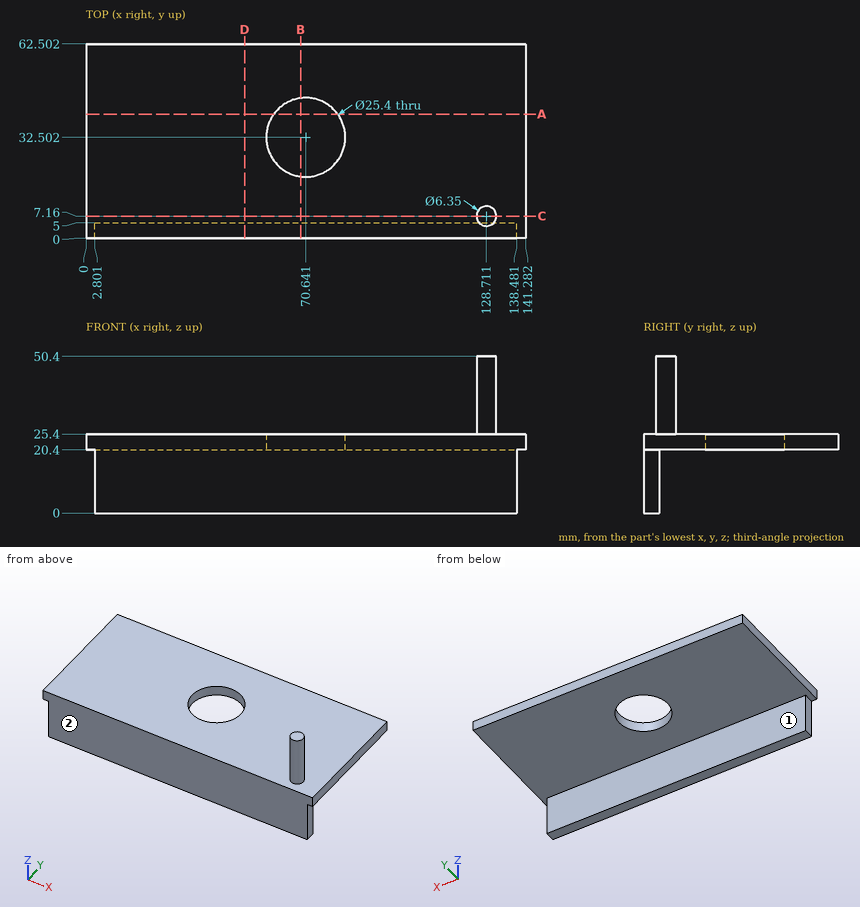
Design review of the part shown in the three views and the two pictorial views. Dimensions are in mm from the part's minimum x, y and z. A direction names the side the tool comes from. Round coordinates to 2 decimals unless told otherwise and drop trailing zeros. Order: outer loops, then holes, each group sorted by start corner. A loop starts at its lowest first (then second) coordinate and runs counter-clockwise, first axis right, second up.
Q1. Insertion check: P1, Ø6, axis at x = 41.5, z = 8, coming from the +Y side; P2, Ø1.5, axis at x = 45, y = 11.5, coming from the -Z side; P3, Ø5, axis at y = 22, z = 29.5, coming from the +X side; P4, Ø1, axis at x = 103, y = 35.5, coming from the +Z side. Each pin has a flat end and moves straight along its axis. Give the tip position at first contact, or say it passes through.
Findings below:
P1: stops at y = 5
P2: stops at z = 20.4
P3: passes through
P4: stops at z = 25.4
Q2. Machinability: for the marked faces 1 and 2, which of the approach directions +Z, -Z, +X, -X, +Y, -Y give a long, thin tool a straight path to every point of the face, cutting with its end or side? Answer none if there is none.
Findings below:
face 1: -Z, +X, -X, +Y
face 2: +Z, -Z, +X, -X, -Y
Q3. Wall thickness on line 1 (Z direction, x = 60.5, y = 41.5); line 2 (Y direction, x = 131.5, z = 15.5); line 3 (X direction, y = 24, z = 22.5) (1 decimal): over which ranges is each line inside the solid? List them lowest first.
Findings below:
line 1: z = 20.4 to 25.4
line 2: y = 0 to 5
line 3: x = 0 to 61.2, 80.1 to 141.3
Q4. We need section A-A, the plane y = 40. Give the boundary of the cut face in (x, z), plus the area to 3 significant figures.
Findings below:
outline: (0, 20.4) - (60.39, 20.4) - (60.39, 25.4) - (0, 25.4) - close; (80.89, 20.4) - (141.28, 20.4) - (141.28, 25.4) - (80.89, 25.4) - close
area: 604 mm2
Q5. We need section B-B, the plane x = 69. Give the boundary of the cut face in (y, z).
Findings below:
outline: (0, 0) - (5, 0) - (5, 20.4) - (19.91, 20.4) - (19.91, 25.4) - (0, 25.4) - close; (45.1, 20.4) - (62.5, 20.4) - (62.5, 25.4) - (45.1, 25.4) - close
Q6. We need section D-D, the plane x = 51. Give the boundary of the cut face in (y, z).
Findings below:
outline: (0, 0) - (5, 0) - (5, 20.4) - (62.5, 20.4) - (62.5, 25.4) - (0, 25.4) - close
Q7. We need section C-C, the plane y = 7.16. Give the boundary of the cut face in (x, z).
Findings below:
outline: (0, 20.4) - (141.28, 20.4) - (141.28, 25.4) - (131.89, 25.4) - (131.89, 50.4) - (125.54, 50.4) - (125.54, 25.4) - (0, 25.4) - close
